from build123d import *

# Parameters (mm, degrees)
BOSS_EXTRUDE1_DEPTH      = 10
BOSS_EXTRUDE1_DEPTH_BACK = 304.8
SKETCH4_R                = 2.585
CUT_EXTRUDE1_DEPTH       = 313.894614847


with BuildPart() as part:
    # Sketch3 → Boss-Extrude1 (new, two sides: drawn at the far end of the back side and taken through both)
    with BuildSketch(Plane.XY.offset(-BOSS_EXTRUDE1_DEPTH_BACK)):
        Polygon((-50, 0), (0, 0), (0, 50), (-3, 50), (-3, 3), (-50, 3), align=None)
    extrude(amount=BOSS_EXTRUDE1_DEPTH + BOSS_EXTRUDE1_DEPTH_BACK)

    # Sketch4 → Cut-Extrude1 (cut, through all)
    with BuildSketch(Plane(origin=(0, 0, 0), x_dir=(1, 0, 0), z_dir=(0, 1, 0))):
        with Locations(Location((-37, 156.19, 0), (0, 0, 180))):
            Circle(SKETCH4_R)
        with Locations(Location((-16, 156.19, 0), (0, 0, 90))):
            Circle(SKETCH4_R)
        with Locations(Location((-37, 184.19, 0), (0, 0, 180))):
            Circle(SKETCH4_R)
        with Locations(Location((-16, 184.19, 0), (0, 0, 90))):
            Circle(SKETCH4_R)
        with Locations(Location((-37, 110.61, 0), (0, 0, 90))):
            Circle(SKETCH4_R)
        with Locations(Location((-16, 110.61, 0), (0, 0, 180))):
            Circle(SKETCH4_R)
        with Locations(Location((-16, 138.61, 0), (0, 0, 180))):
            Circle(SKETCH4_R)
        with Locations(Location((-37, 138.61, 0), (0, 0, 90))):
            Circle(SKETCH4_R)
    extrude(amount=CUT_EXTRUDE1_DEPTH, mode=Mode.SUBTRACT)


solid = part.part
Geometry: final body of the model. Coordinates: model frame, mm. A direction names the side the tool comes from. Give positions to 0.01 mm unless a question says otherwise; leave off trailing zeros. Write each loop counter-clockwise with the first axis right and the second up, starting at its lowest first coordinate (ties: lowest second). Pieces come first, ordered by that corner, then holes. Notation, with made-up numbers: (75, 44) - (128, 44) arc R33 cw to (128, 82) - close; hole circle Ø10 at (81, 5.25). An arc over 180 degrees is marked (long way). Return JSON: item names as keys, results as strings. Group by question number.
1) Section C-C on z = -55. Return the cut outline in (x, y), plus the area to 3 significant figures.
2) Mould query, pull axis Z, two halves, no side actions, for faces 3 (the cylindrical face through (-15.44, 1.479, -141.134)), 4 (the flat face through (-25, 0, -150)). Classes: released by +Z, released by -Z, zero draft, split by the parting line, or undercut.
3) Section B-B on z = -184.19. Return the cut outline in (x, y) (3 decimals), plus the area to 3 significant figures.
4) Set-up query: faces 1 (the flat face through (-26, 3, -150)), 2 (the cylindrical face through (-16.776, 1.479, -158.656)). Return all of +Z, -Z, +X, -X, +Y, -Y with unobstructed straight access to the full face (end or side cutting, diameter ignored); none if empty.
5) First-contact query: P1, Ø8, axis at y = 20.5, z = -49.5, coming from the +X side; P2, Ø3, axis at x = -44.5, z = -103.5, coming from the +Y side; P3, Ø14, axis at y = 17, z = -75, coming from the -X side. Flat tips, straight axial feed; report the tip coordinate or a pass-through.
6) Line query: line 1 (X direction, y = 1, z = -156); line 2 (Z direction, x = -37, y = 2) (3 decimals); line 3 (Y direction, x = -47, z = -161). Output: solid intervals per line, ascending.
7) Section D-D on x = -6. Return the cut outline in (y, z), plus the area to 3 significant figures.
8) Section A-A on x = -37. Return the cut outline in (y, z) (3 decimals).
Filled in:
{
 "1": {"outline": "(-50, 0) - (0, 0) - (0, 50) - (-3, 50) - (-3, 3) - (-50, 3) - close", "area": "291 mm^2"},
 "2": {"face 3": "undercut", "face 4": "zero draft"},
 "3": {"outline": "(-50, 0) - (-39.585, 0) - (-39.585, 3) - (-50, 3) - close; (-34.415, 0) - (-18.585, 0) - (-18.585, 3) - (-34.415, 3) - close; (-13.415, 0) - (0, 0) - (0, 50) - (-3, 50) - (-3, 3) - (-13.415, 3) - close", "area": "260 mm^2"},
 "4": {"face 1": "+Z, -Z, -X, +Y", "face 2": "+Y, -Y"},
 "5": {"P1": "stops at x = 0", "P2": "stops at y = 3", "P3": "stops at x = -3"},
 "6": {"line 1": "x = -50 to -39.58, -34.42 to -18.58, -13.42 to 0", "line 2": "z = -304.8 to -186.775, -181.605 to -158.775, -153.605 to -141.195, -136.025 to -113.195, -108.025 to 10", "line 3": "y = 0 to 3"},
 "7": {"outline": "(0, -304.8) - (3, -304.8) - (3, 10) - (0, 10) - close", "area": "944 mm^2"},
 "8": {"outline": "(0, -304.8) - (3, -304.8) - (3, -186.775) - (0, -186.775) - close; (0, -181.605) - (3, -181.605) - (3, -158.775) - (0, -158.775) - close; (0, -153.605) - (3, -153.605) - (3, -141.195) - (0, -141.195) - close; (0, -136.025) - (3, -136.025) - (3, -113.195) - (0, -113.195) - close; (0, -108.025) - (3, -108.025) - (3, 10) - (0, 10) - close"}
}
